Geometry: see drawing. Coordinates: mm, zero at the bounding-box minimum. A direction names the side the tool comes from. Coordinates: 2 decimals unless noted, no trailing zeros. Write each loop counter-clockwise with the first axis right and the second up, starting at its lowest first coordinate (ties: lowest second). Pieces come first, ordered by that corner, then holes. Notation, with made-up numbers: (0.5, 23.5) -> (31.5, 23.5) arc R32 ccw to (31.5, 52.5) -> close; hole circle Ø5 at (86, 81). An arc over 180 degrees is marked (long way). Use one line per item in the form item = value. Start each with the question number.
(1) Cut plane C-C on y = 12.5. Return the cut outline in (x, z), plus the area to 3 significant figures.
(2) Cut plane B-B on x = 23. Return the cut outline in (y, z), plus the area to 3 significant figures.
(3) First-contact query: pin 1 (2 mm diameter, centred on x = 20.5, z = 18, fed in from -Y); pin 2 (3.5 mm diameter, centred on y = 10, z = 37, fed in from -X); pin 3 (3 mm diameter, centred on x = 23, y = 9, fed in from +Z). Flat tips, straight axial feed; report the tip coordinate or a pass-through.
(4) Ray query, line 1 along Y through (x, z) = (23, 84); line 2 along Y through (x, z) = (15.5, 4); line 3 along Z through (x, y) = (23, 19.5). Return the intervals inside material, ascending.
(5) Pull-direction query (Z, two-part tool) for the marked faces 5, 6, 7 and 8; classes: released by +Z, released by -Z, zero draft, split by the parting line, or undercut.
(6) Cut plane A-A on y = 19. Return the cut outline in (x, z), plus the area to 3 significant figures.
(7) Set-up query: the marked faces 1, 2, 3 and 4. Return all of +Z, -Z, +X, -X, +Y, -Y with unobstructed straight access to the full face (end or side cutting, diameter ignored); none if empty.
(8) Cut plane D-D on x = 19. Return the cut outline in (y, z).
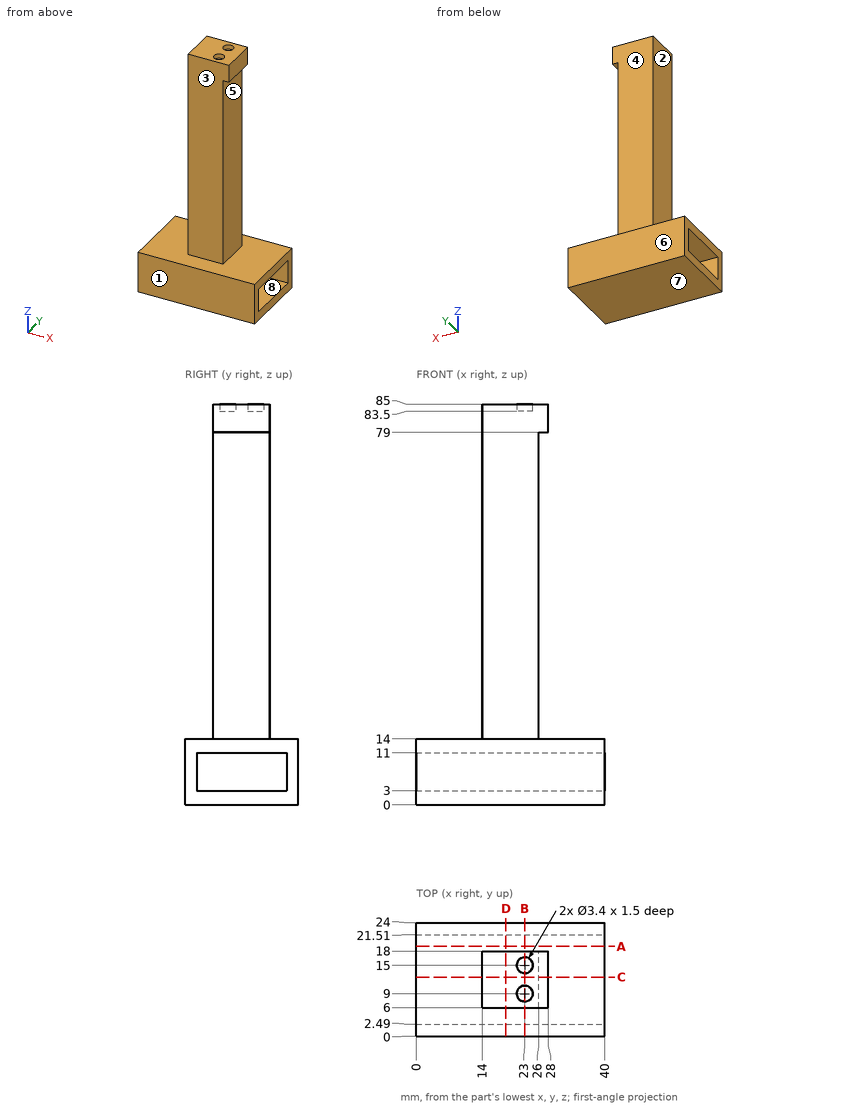
Values:
q1.outline = (0, 0) -> (40, 0) -> (40, 3) -> (0, 3) -> close; (0, 11) -> (40, 11) -> (40, 14) -> (26, 14) -> (26, 79) -> (28, 79) -> (28, 85) -> (14, 85) -> (14, 14) -> (0, 14) -> close
q1.area = 1,100 mm2
q2.outline = (0, 0) -> (24, 0) -> (24, 14) -> (18, 14) -> (18, 85) -> (16.7, 85) -> (16.7, 83.5) -> (13.3, 83.5) -> (13.3, 85) -> (10.7, 85) -> (10.7, 83.5) -> (7.3, 83.5) -> (7.3, 85) -> (6, 85) -> (6, 14) -> (0, 14) -> close; hole (2.49, 3) -> (21.51, 3) -> (21.51, 11) -> (2.49, 11) -> close
q2.area = 1,030 mm2
q3.pin_1 = 6
q3.pin_2 = 14
q3.pin_3 = 83.5
q4.line_1 = 6 to 7.3, 10.7 to 13.3, 16.7 to 18
q4.line_2 = 0 to 2.49, 21.51 to 24
q4.line_3 = 0 to 3, 11 to 14
q5.face_5 = undercut
q5.face_6 = zero draft
q5.face_7 = released by -Z
q5.face_8 = undercut
q6.outline = (0, 0) -> (40, 0) -> (40, 3) -> (0, 3) -> close; (0, 11) -> (40, 11) -> (40, 14) -> (0, 14) -> close
q6.area = 240 mm2
q7.face_1 = +Z, -Z, +X, -X, -Y
q7.face_2 = +Z, -X, +Y, -Y
q7.face_3 = +Z, +X, -X, -Y
q7.face_4 = +Z, +X, -X, +Y
q8.outline = (0, 0) -> (24, 0) -> (24, 14) -> (18, 14) -> (18, 85) -> (6, 85) -> (6, 14) -> (0, 14) -> close; hole (2.49, 3) -> (21.51, 3) -> (21.51, 11) -> (2.49, 11) -> close
